The model under review builds one solid part; all positions refer to its coordinate system, in mm. A direction names the side the tool comes from. Give positions to 0.01 mm unless a question says otherwise; leave off trailing zeros. Loops run counter-clockwise (first coordinate to the right, second up) from the corner with the lowest first, then second, coordinate; pieces in that order, holes last. Notation, with made-up numbers: (-19, -13.5) - (4, -13.5) arc R6 ccw to (4, -3.5) - close; hole circle Ø5 at (51, -13). An arc over 180 degrees is marked (long way). Answer as a JSON object with one key per item and string values.
from build123d import *

# Parameters (mm, degrees)
SKETCH1_W           = 40
SKETCH1_H           = 30
BOSS_EXTRUDE1_DEPTH = 7
SKETCH2_W           = 20
SKETCH2_H           = 20
CUT_EXTRUDE1_DEPTH  = 4
SKETCH3_W           = 4
SKETCH3_H           = 12
CUT_EXTRUDE2_DEPTH  = 26
SKETCH4_R           = 1.25
CUT_EXTRUDE3_DEPTH  = 8
SKETCH5_W           = 24
SKETCH5_H           = 7
BOSS_EXTRUDE2_DEPTH = 7
SKETCH6_R           = 1.75
CUT_EXTRUDE4_DEPTH  = 8


with BuildPart() as part:
    # Sketch1 → Boss-Extrude1 (new body)
    with BuildSketch(Plane.XY):
        with Locations((20, 15)):
            Rectangle(SKETCH1_W, SKETCH1_H)
    extrude(amount=BOSS_EXTRUDE1_DEPTH)

    # Sketch2 → Cut-Extrude1 (cut)
    with BuildSketch(Plane.XY.offset(7)):
        with Locations((20, 15)):
            Rectangle(SKETCH2_W, SKETCH2_H)
    extrude(amount=-CUT_EXTRUDE1_DEPTH, mode=Mode.SUBTRACT)

    # Sketch3 → Cut-Extrude2 (cut)
    with BuildSketch(Plane.ZY):
        with Locations((5, 15)):
            Rectangle(SKETCH3_W, SKETCH3_H)
    extrude(amount=-CUT_EXTRUDE2_DEPTH, mode=Mode.SUBTRACT)

    # Sketch4 → Cut-Extrude3 (cut, through all)
    with BuildSketch(Plane.XY.offset(7)):
        with Locations((2, 28)):
            Circle(SKETCH4_R)
        with Locations((38, 28)):
            Circle(SKETCH4_R)
        with Locations((38, 2)):
            Circle(SKETCH4_R)
        with Locations((2, 2)):
            Circle(SKETCH4_R)
    extrude(amount=-CUT_EXTRUDE3_DEPTH, mode=Mode.SUBTRACT)

    # Sketch5 → Boss-Extrude2 (add)
    with BuildSketch(Plane.XY.offset(7)):
        with Locations((20, 33.5)):
            Rectangle(SKETCH5_W, SKETCH5_H)
        with Locations((20, -3.5)):
            Rectangle(SKETCH5_W, SKETCH5_H)
    extrude(amount=-BOSS_EXTRUDE2_DEPTH)

    # Sketch6 → Cut-Extrude4 (cut, through all)
    with BuildSketch(Plane.XY.offset(7)):
        with Locations((20, -2)):
            Circle(SKETCH6_R)
        with Locations((20, 32)):
            Circle(SKETCH6_R)
    extrude(amount=-CUT_EXTRUDE4_DEPTH, mode=Mode.SUBTRACT)


solid = part.part
Q1. Clearance check with flat-ended pins moving along their axes: pin 1 Ø2 at (x, z) = (3.5, 4) entering from -Y; pin 2 Ø3.5 at (y, z) = (-2.5, 5) entering from +X; pin 3 Ø12 at (x, y) = (21, 14.5) entering from +Z; pin 4 Ø2 at (x, y) = (20, 32) entering from -Z. State where each tip first meets the part, or that it passes through.
Results:
{"pin 1": "stops at y = 0", "pin 2": "stops at x = 32", "pin 3": "stops at z = 3", "pin 4": "passes through"}
Q2. For faces 1 (the face through (5, 21, 5)), 2 (the face through (10, 23, 5)), 3 (the face through (4, 30, 3)), list the 3-axis set-ups (+Z, -Z, +X, -X, +Y, -Y) from which the entire face can be reached by the end or side of a thin tool; tool diameter is ignored.
Results:
{"face 1": "+Z, -X", "face 2": "+Z", "face 3": "+Z, -Z, -X, +Y"}
Q3. Consider section B-B, the plane x = 2. State the section outline as (y, z) points, plus the area to 3 significant figures.
Results:
{"outline": "(0, 0) - (0.75, 0) - (0.75, 7) - (0, 7) - close; (3.25, 0) - (26.75, 0) - (26.75, 7) - (21, 7) - (21, 3) - (9, 3) - (9, 7) - (3.25, 7) - close; (29.25, 0) - (30, 0) - (30, 7) - (29.25, 7) - close", "area": "127 mm^2"}
Q4. To check wall thickness, follow probe 1 along Y at (x, z) = (38, 2); probe 2 along Y at (x, z) = (20, 5.75); probe 3 along Y at (x, z) = (2, 5.25). State the ranges of each line that lie inside material, in increasing order. Write a range as [from, to].
Results:
{"probe 1": "y = [0, 0.75], [3.25, 26.75], [29.25, 30]", "probe 2": "y = [-7, -3.75], [-0.25, 5], [25, 30.25], [33.75, 37]", "probe 3": "y = [0, 0.75], [3.25, 9], [21, 26.75], [29.25, 30]"}
Q5. The part is to be moulded in two halves that separate along Y. For faces 4 (the face through (40, 15, 3)), 5 (the face through (4, 0, 3)), 6 (the face through (36.75, 2.05, 3.55)), 7 (the face through (36, 30, 3)), say which applies: +Y half, -Y half, draft (parallel to the pull), parting line (faces both ways), or undercut.
Results:
{"face 4": "draft", "face 5": "-Y half", "face 6": "undercut", "face 7": "+Y half"}
Q6. Consider section A-A, the plane y = -2. State the section outline as (x, z) points.
Results:
{"outline": "(8, 0) - (18.25, 0) - (18.25, 7) - (8, 7) - close; (21.75, 0) - (32, 0) - (32, 7) - (21.75, 7) - close"}
Q7. Consider section C-C, the plane z = 1. State the section outline as (x, y) points.
Results:
{"outline": "(0, 0) - (8, 0) - (8, -7) - (32, -7) - (32, 0) - (40, 0) - (40, 30) - (32, 30) - (32, 37) - (8, 37) - (8, 30) - (0, 30) - close; hole circle Ø2.5 at (2, 2); hole circle Ø2.5 at (2, 28); hole circle Ø3.5 at (20, -2); hole circle Ø3.5 at (20, 32); hole circle Ø2.5 at (38, 2); hole circle Ø2.5 at (38, 28)"}
Q8. Consider section D-D, the plane y = 28. State the section outline as (x, z) points.
Results:
{"outline": "(0, 0) - (0.75, 0) - (0.75, 7) - (0, 7) - close; (3.25, 0) - (36.75, 0) - (36.75, 7) - (3.25, 7) - close; (39.25, 0) - (40, 0) - (40, 7) - (39.25, 7) - close"}
